The listing builds one solid part. Answer for the finished solid, in the listing's coordinates (mm). Round coordinates to 2 decimals unless told otherwise and drop trailing zeros. Loops run counter-clockwise (first coordinate to the right, second up) from the corner with the lowest first, then second, coordinate; pieces in that order, holes last. Notation, with made-up numbers: M 10,8 L 66,8 A23 cw 66,30 Z; hole C -17.75,-23.5 d10. An arc over 180 degrees is marked long. Answer as a JSON object with one key per item and string values.
```python
from build123d import *

# Parameters (mm, degrees)
BOSS_EXTRUDE1_DEPTH = 0.75
FILLET1_R           = 2


with BuildPart() as part:
    # Sketch1 → Boss-Extrude1 (new body)
    with BuildSketch(Plane.XY):
        Polygon((-152.5, -152.5), (-50, -152.5), (-40, -162.5), (40, -162.5), (50, -152.5), (152.5, -152.5), (152.5, 152.5), (-152.5, 152.5), align=None)
    extrude(amount=BOSS_EXTRUDE1_DEPTH)

    # Fillet1
    fillet1_edges = [part.edges().sort_by_distance(p)[0] for p in [
        (152.5, -152.5, 0.375),
        (50, -152.5, 0.375),
        (40, -162.5, 0.375),
        (-40, -162.5, 0.375),
        (-50, -152.5, 0.375),
        (-152.5, -152.5, 0.375),
        (-152.5, 152.5, 0.375),
        (152.5, 152.5, 0.375),
    ]]
    fillet(fillet1_edges, radius=FILLET1_R)


solid = part.part
```
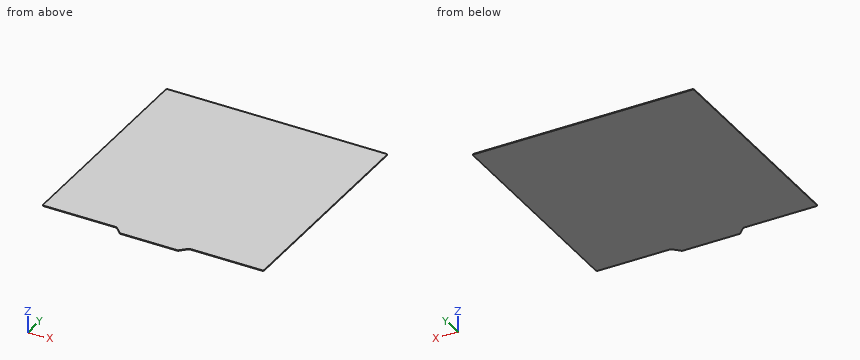
Item 1: The part is cut by section A-A (z = 0.15). Give the vertices of the cut face in (x, y).
Values follow:
{"outline": "M -152.5,-150.5 A2 ccw -150.5,-152.5 L -50.83,-152.5 A2 cw -49.41,-153.09 L -40.59,-161.91 A2 ccw -39.17,-162.5 L 39.17,-162.5 A2 ccw 40.59,-161.91 L 49.41,-153.09 A2 cw 50.83,-152.5 L 150.5,-152.5 A2 ccw 152.5,-150.5 L 152.5,150.5 A2 ccw 150.5,152.5 L -150.5,152.5 A2 ccw -152.5,150.5 Z"}
Item 2: The part is cut by section B-B (x = -105.5). Give the vertices of the cut face in (y, z), then the cut area to 3 significant figures.
Values follow:
{"outline": "M -152.5,0 L 152.5,0 L 152.5,0.75 L -152.5,0.75 Z", "area": "229 mm^2"}
Item 3: A flat-ended cylindrical pin translates along its axis: P1, Ø1, axis at x = -61.5, y = 17.5, coming from the -Z side. Find the tip coordinate at first contact, or state that the pin passes through.
Values follow:
{"P1": "z = 0"}
Item 4: A straight line is drawn through the part: line 1 (Y direction, x = -110, z = 0.4). Find the intervals that lie inside material, in ascending order.
Values follow:
{"line 1": "-152.5 to 152.5"}
